Here's how the part is built. I have some questions about the finished solid (model axes, mm). Face numbers are marked on the shaded views. A direction names the side the tool comes from. Round coordinates to 2 decimals unless told otherwise and drop trailing zeros. Write each loop counter-clockwise with the first axis right and the second up, starting at its lowest first coordinate (ties: lowest second). Pieces come first, ordered by that corner, then holes. Notation, with made-up numbers: (49.5, 40) -> (104.5, 40) arc R17 ccw to (104.5, 46) -> close; hole circle Ø1 at (65, 67). An arc over 180 degrees is marked (long way). Put each result on its own line as item: value. Start each with the question number.
1. For pin 1 (2 mm diameter, centred on x = -16.5, z = 19, fed in from -Y); pin 2 (2 mm diameter, centred on y = 40, z = 27, fed in from +X); pin 3 (6 mm diameter, centred on y = 14.5, z = 23, fed in from -X), each with a flat end and sliding along its axis, tell me the tip position at first contact or that it passes through.
2. I need wall thicknesses on probe 1 along Y at (x, z) = (0, 7); probe 2 along X at (y, z) = (10.5, 8.5); probe 3 along Y at (x, z) = (-6, 9). Which ranges of each line are inside material? Lowest first, please. Write a range as from..to.
3. Suppose I cut it at A-A (y = 0). Please give me the cut outline in (x, z).
4. Which directions (+Z, -Z, +X, -X, +Y, -Y) give clear straight access to the entire face, cutting with the end or side of a thin tool? Please do the marked faces 5 and 6.
5. We'd pull the mould along X, two halves only. Please class the marked faces 1, 2, 3 and 4: +X half, -X half, draft (parallel to the pull), parting line (faces both ways), or undercut.
6. Suppose I cut it at C-C (z = 2.25). Please give me the cut outline in (x, y), then the cut area to 3 significant figures.
7. Suppose I cut it at D-D (x = -38). Please give me the cut outline in (y, z).
```python
from build123d import *

# Parameters (mm, degrees)
SKETCH1_R           = 50
BOSS_EXTRUDE1_DEPTH = 30
SKETCH2_R           = 2.5
CUT_EXTRUDE1_DEPTH  = 31
SHELL1_T            = -10


with BuildPart() as part:
    # Sketch1 → Boss-Extrude1 (new body)
    with BuildSketch(Plane.XY):
        Circle(SKETCH1_R)
    extrude(amount=BOSS_EXTRUDE1_DEPTH)

    # Sketch2 → Cut-Extrude1 (cut, through all)
    with BuildSketch(Plane(origin=(0, 0, 0), x_dir=(-1, 0, 0), z_dir=(0, 0, -1))):
        Circle(SKETCH2_R)
    extrude(amount=-CUT_EXTRUDE1_DEPTH, mode=Mode.SUBTRACT)

    # Shell1
    shell1_openings = [part.faces().sort_by_distance(p)[0] for p in [
        (-2.5, 0, 0),
    ]]
    offset(amount=SHELL1_T, openings=shell1_openings, kind=Kind.INTERSECTION)


solid = part.part
```
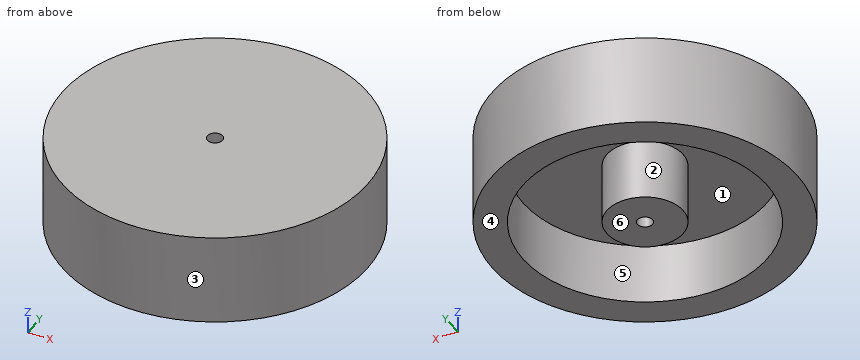
Verdict:
1. pin 1: stops at y = -47.54
1. pin 2: stops at x = 31.29
1. pin 3: stops at x = -48.66
2. probe 1: y = -50..-40, -12.5..-2.5, 2.5..12.5, 40..50
2. probe 2: x = -48.89..-38.6, -6.78..6.78, 38.6..48.89
2. probe 3: y = -49.64..-39.55, -10.97..10.97, 39.55..49.64
3. outline: (-50, 0) -> (-40, 0) -> (-40, 20) -> (-12.5, 20) -> (-12.5, 0) -> (-2.5, 0) -> (-2.5, 30) -> (-50, 30) -> close; (2.5, 0) -> (12.5, 0) -> (12.5, 20) -> (40, 20) -> (40, 0) -> (50, 0) -> (50, 30) -> (2.5, 30) -> close
4. face 5: -Z
4. face 6: -Z, +X, -X, +Y, -Y
5. face 1: undercut
5. face 2: undercut
5. face 3: parting line
5. face 4: draft
6. outline: circle Ø100 at (0, 0); circle Ø25 at (0, 0); hole circle Ø80 at (0, 0); hole circle Ø5 at (0, 0)
6. area: 3,300 mm^2
7. outline: (-32.5, 0) -> (-12.49, 0) -> (-12.49, 20) -> (12.49, 20) -> (12.49, 0) -> (32.5, 0) -> (32.5, 30) -> (-32.5, 30) -> close
